from build123d import *


with BuildPart() as f1:
    # F0 (on Front) → F1 (revolve)
    with BuildSketch(Plane.XZ):
        with BuildLine():
            Line((-2.5, 0), (0, 0))
            Line((0, 0), (0, 5.499265))
            ThreePointArc((0, 5.499265), (-2.090062, 5.409453), (-3.974026, 4.5))
            Line((-3.974026, 4.5), (-3.974026, 4))
            Line((-3.974026, 4), (-2.5, 4))
            Line((-2.5, 4), (-2.5, 0))
        make_face()
    revolve(axis=Axis((0, 0, 2.749633), (0, 0, 1)))

    # F2: F1 across face


with BuildPart() as f1_1:
    add(f1.part)
    add(f1.part.mirror(Plane(origin=(0, 0, 0), x_dir=(1, 0, 0), z_dir=(0, 0, -1))))


solid = f1_1.part
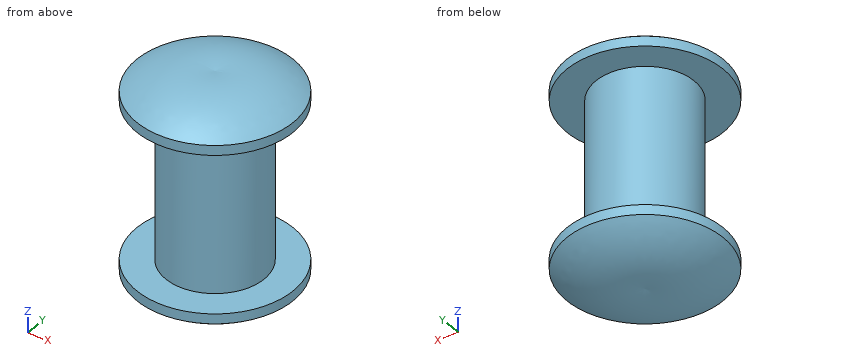
Can you work these out from the model? Positions are in its coordinate system, mm. Coordinates: 2 decimals unless noted, no trailing zeros. Order: outer loops, then holes, each group sorted by start corner. A loop starts at its lowest first (then second) coordinate and runs counter-clockwise, first axis right, second up. Notation, with made-up numbers: M 31,-1 L 74,-1 A17 cw 74,24 Z; hole C 73.5,-36.5 d2. An arc over 180 degrees is marked long. Answer as CSV lines item,"result".
(1) Please list where these lines run through material, in increasing order: L1, parallel to Z at x = -2.25, y = 3; L2, parallel to Z at x = -3, y = -2; L3, parallel to Y at x = -1.5, z = 3.5.
Geometry check:
L1,"-4.66 to -4, 4 to 4.66"
L2,"-4.76 to -4, 4 to 4.76"
L3,"-2 to 2"
(2) I'm going to push flat-ended pins straight in: pin 1 (1.5 mm diameter, centred on x = -2.5, y = -1.5, fed in from +Z); pin 2 (1.5 mm diameter, centred on y = 0.5, z = 1.5, fed in from +X); pin 3 (1 mm diameter, centred on x = -2.5, z = -1, fed in from +Y). Where does each tip first touch, or does it pass through?
Geometry check:
pin 1,"z = 5.39"
pin 2,"x = 2.5"
pin 3,"y = 1.5"
(3) Suppose I cut it at A-A on z = -0.25. Please give me the cut outline in (x, y), plus the area to 3 significant figures.
Geometry check:
outline,"C 0,0 d5"
area,"19.6 mm^2"
